```python
from build123d import *

# Parameters (mm, degrees)
SKETCH_R              = 25
PAD_DEPTH             = 16
PAD001_DEPTH          = 16
POLARPATTERN_COUNT    = 12
POCKET_DEPTH          = 16.001
POCKET001_DEPTH       = 275.369464
POLARPATTERN001_COUNT = 3


with BuildPart() as part:
    # Sketch → Pad (new body)
    with BuildSketch(Plane.XY):
        Circle(SKETCH_R)
    extrude(amount=PAD_DEPTH)

    # Sketch002 → Pad001 (join)
    with BuildSketch(Plane.XY):
        with BuildLine():
            Line((15.28351, 1), (45.48901, 1))
            ThreePointArc((45.48901, -1), (45.5, 0), (45.48901, 1))
            Line((15.28351, -1), (45.48901, -1))
            Line((15.28351, 1), (15.28351, -1))
        make_face()
    pad001 = extrude(amount=PAD001_DEPTH)

    # PolarPattern: Pad001 ×12 about axis
    polarpattern_axis = Axis((0, 0, 0), (0, 0, 1))
    for i in range(1, POLARPATTERN_COUNT):
        add(pad001.rotate(polarpattern_axis, i * 360 / POLARPATTERN_COUNT))

    # Sketch003 → Pocket (cut, through all)
    with BuildSketch(Plane.XY):
        Polygon((-5.3, 0), (-2.65, -4.589935), (2.65, -4.589935), (5.3, 0), (2.65, 4.589935), (-2.65, 4.589935), align=None)
    extrude(amount=POCKET_DEPTH, mode=Mode.SUBTRACT)

    # Sketch004 → Pocket001 (cut, through all)
    with BuildSketch(Plane.XY):
        with BuildLine():
            Line((-1.5, 22.951035), (-1.5, 8.87412))
            ThreePointArc((-1.5, 8.87412), (-7.794229, 4.5), (-8.435213, -3.138022))
            Line((-8.435213, -3.138022), (-20.626179, -10.176479))
            ThreePointArc((-1.5, 22.951035), (-19.918584, 11.5), (-20.626179, -10.176479))
        make_face()
    pocket001 = extrude(amount=POCKET001_DEPTH, mode=Mode.SUBTRACT)

    # PolarPattern001: Pocket001 ×3 about axis
    polarpattern001_axis = Axis((0, 0, 0), (0, 0, 1))
    for i in range(1, POLARPATTERN001_COUNT):
        add(pocket001.rotate(polarpattern001_axis, i * 360 / POLARPATTERN001_COUNT), mode=Mode.SUBTRACT)


solid = part.part
```
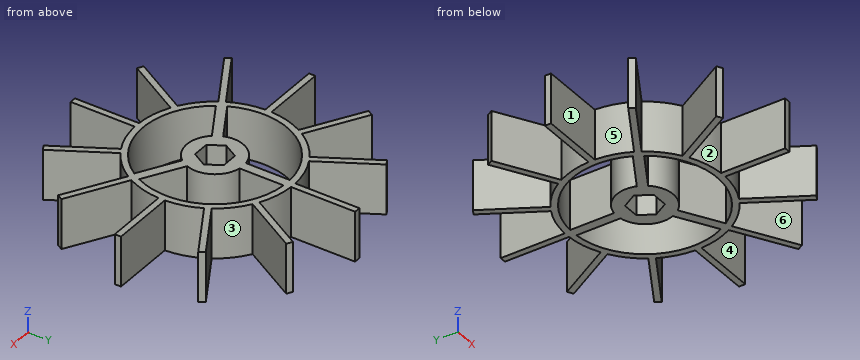
Verification items for the finished model (mm, model axes). Face numbers are marked on the shaded views. A direction names the side the tool comes from. Coordinates: 2 decimals unless noted, no trailing zeros. Loops run counter-clockwise (first coordinate to the right, second up) from the corner with the lowest first, then second, coordinate; pieces in that order, holes last. Notation, with made-up numbers: (-15.5, -40) -> (-0.5, -40) arc R13 ccw to (-0.5, -32) -> close; hole circle Ø10 at (-4, -6). An arc over 180 degrees is marked (long way). Answer in a Markdown table with one row per item.
1) Section check D-D (x = 37). Record the cut outline in (y, z), and give its area (3 significant figures).
The answers:
| item | result |
|---|---|
| outline | (-22.52, 0) -> (-20.21, 0) -> (-20.21, 16) -> (-22.52, 16) -> close; (-1, 0) -> (1, 0) -> (1, 16) -> (-1, 16) -> close; (20.21, 0) -> (22.52, 0) -> (22.52, 16) -> (20.21, 16) -> close |
| area | 106 mm2 |
2) Access from +Z, -Z, +X, -X, +Y, -Y to the whole of each face (thin tool, end or side, straight path). Record for the marked faces 1, 2 and 3.
The answers:
| item | result |
|---|---|
| face 1 | +Z, -Z, -X |
| face 2 | +Z, -Z, -Y |
| face 3 | +Z, -Z |
3) Section check C-C (y = 16). Record the cut outline in (x, z).
The answers:
| item | result |
|---|---|
| outline | (-29.71, 0) -> (-25.71, 0) -> (-25.71, 16) -> (-29.71, 16) -> close; (-19.21, 0) -> (-16.52, 0) -> (-16.52, 16) -> (-19.21, 16) -> close; (-1.5, 0) -> (1.5, 0) -> (1.5, 16) -> (-1.5, 16) -> close; (16.52, 0) -> (19.21, 0) -> (19.21, 16) -> (16.52, 16) -> close; (25.71, 0) -> (29.71, 0) -> (29.71, 16) -> (25.71, 16) -> close |
4) Section check B-B (x = -4). Record the cut outline in (y, z).
The answers:
| item | result |
|---|---|
| outline | (-24.68, 0) -> (-22.65, 0) -> (-22.65, 16) -> (-24.68, 16) -> close; (-8.06, 0) -> (-2.25, 0) -> (-2.25, 16) -> (-8.06, 16) -> close; (2.25, 0) -> (8.06, 0) -> (8.06, 16) -> (2.25, 16) -> close; (22.65, 0) -> (24.68, 0) -> (24.68, 16) -> (22.65, 16) -> close |
5) Depth check by flat-ended pin: P1, Ø5, axis at y = 31, z = 9.5, coming from the -X side; P2, Ø3, axis at x = 28.5, y = -12, coming from the -Z side; P3, Ø1, axis at x = 16, z = 5.5, coming from the -Y side; P4, Ø5, axis at x = -31, z = 4, coming from the -Y side. Enter the tip coordinate at first touch or a pass-through.
The answers:
| item | result |
|---|---|
| P1 | stops at x = -20.5 |
| P2 | passes through |
| P3 | stops at y = -30.58 |
| P4 | stops at y = -20.5 |
6) Scan lines: line 1 along Y through (x, z) = (-33, 11.25); line 2 along Y through (x, z) = (-32, 8.5); line 3 along X through (y, z) = (-37, 9). Record each from-to range of solid material in increasing order. Write a range as from..to.
The answers:
| item | result |
|---|---|
| line 1 | y = -20.21..-17.9, -1..1, 17.9..20.21 |
| line 2 | y = -19.63..-17.32, -1..1, 17.32..19.63 |
| line 3 | x = -22.52..-20.21, -1..1, 20.21..22.52 |
7) Section check A-A (y = -15). Record the cut outline in (x, z).
The answers:
| item | result |
|---|---|
| outline | (-27.98, 0) -> (-23.98, 0) -> (-23.98, 16) -> (-27.98, 16) -> close; (-20, 0) -> (-17.44, 0) -> (-17.44, 16) -> (-20, 16) -> close; (17.44, 0) -> (20, 0) -> (20, 16) -> (17.44, 16) -> close; (23.98, 0) -> (27.98, 0) -> (27.98, 16) -> (23.98, 16) -> close |
8) Draft check along X on the marked faces 4, 5 and 6. Enter one of: released by +X, released by -X, zero draft, split by the parting line, or undercut.
The answers:
| item | result |
|---|---|
| face 4 | zero draft |
| face 5 | released by -X |
| face 6 | undercut |
